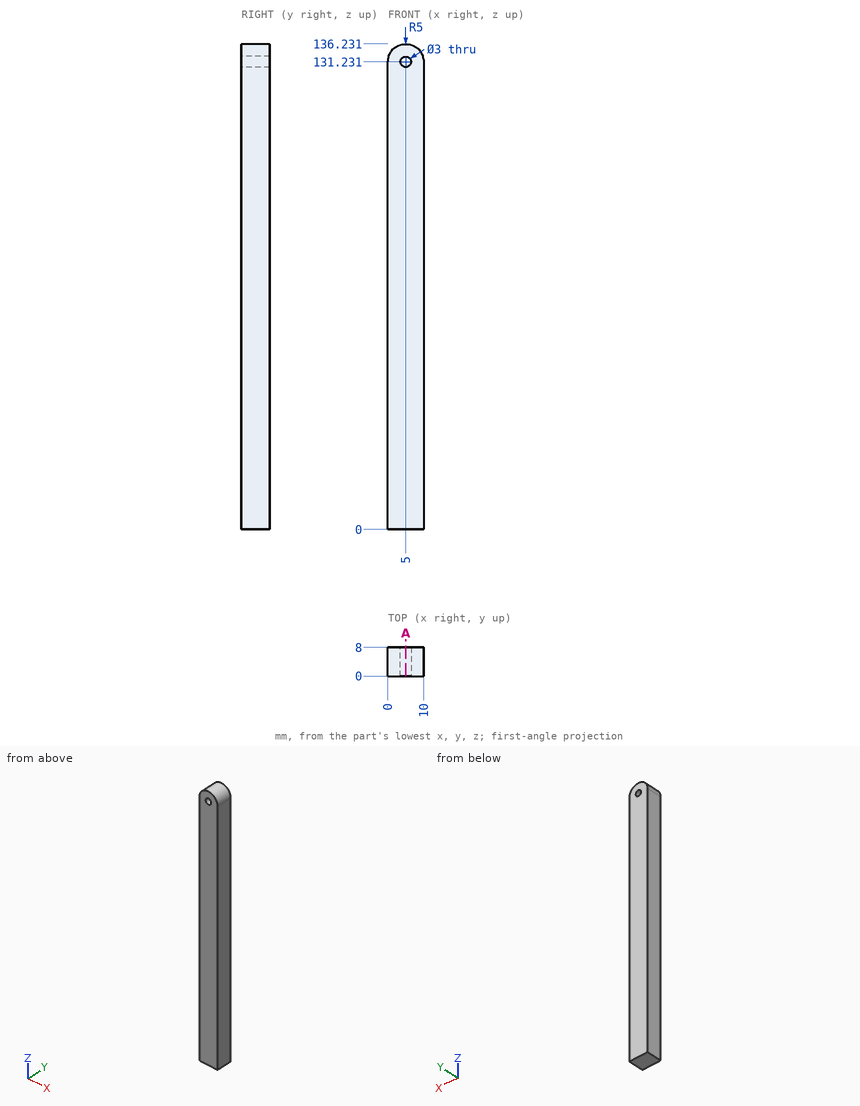
Geometry check sheet. Reference: drawing and pictorial views, mm from the part's lowest x, y, z. Give positions to 0.01 mm unless a question says otherwise; leave off trailing zeros. Loops run counter-clockwise (first coordinate to the right, second up) from the corner with the lowest first, then second, coordinate; pieces in that order, holes last. Notation, with made-up numbers: (25, 77) - (42, 77) arc R17 ccw to (42, 108) - close; hole circle Ø8 at (76, -14). An arc over 180 degrees is marked (long way). Use CSV: the item, a comma, the result in double quotes. Start each with the question number.
Q1. Scan lines: probe 1 along Z at (x, y) = (5, 4.75); probe 2 along Z at (x, y) = (4.75, 1.75) (1 decimal); probe 3 along Z at (x, y) = (2.25, 6). Record each from-to range of solid material in increasing order. Write a range as from..to.
Q2. Go/stop test with flat-tipped pins: pin 1 Ø2 at (x, y) = (7, 2) entering from +Z; pin 2 Ø2 at (x, y) = (8, 6.5) entering from +Z. Record where each tip stops, or that it passes through.
Q3. Section check A-A, the plane x = 5. Record the cut outline in (y, z).
Findings below:
1,probe 1,"z = 0..129.73, 132.73..136.23"
1,probe 2,"z = 0..129.8, 132.7..136.2"
1,probe 3,"z = 0..135.41"
2,pin 1,"stops at z = 136.13"
2,pin 2,"stops at z = 135.81"
3,outline,"(0, 0) - (8, 0) - (8, 129.73) - (0, 129.73) - close; (0, 132.73) - (8, 132.73) - (8, 136.23) - (0, 136.23) - close"
